Build history of the part. All positions in model axes, mm. Face numbers are marked on the shaded views. A direction names the side the tool comes from. Give positions to 0.01 mm unless a question says otherwise; leave off trailing zeros. Order: outer loops, then holes, each group sorted by start corner. A loop starts at its lowest first (then second) coordinate and runs counter-clockwise, first axis right, second up. Notation, with made-up numbers: (-14, 61.25) -> (24, 61.25) arc R18 cw to (24, 93.25) -> close; hole circle Ø2 at (13.25, 27.5). An arc over 180 degrees is marked (long way). Use a Markdown table: item, result. Add a question column.
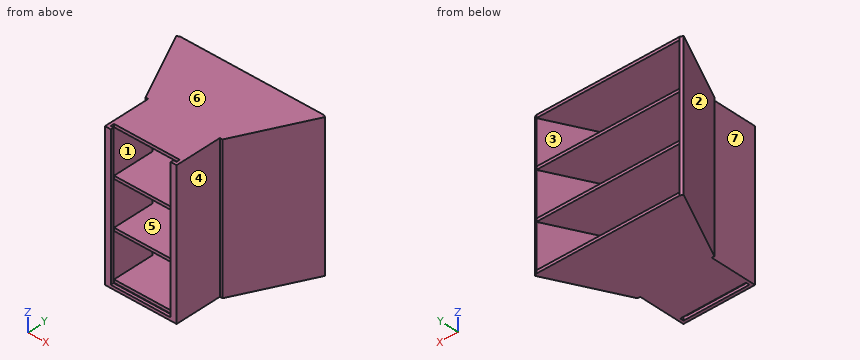
Autodesk Inventor part; units mm, degrees
ref_plane "YZ Plane" through (0, 0, 0) normal (1, 0, 0) x (0, 1, 0)
ref_plane "XZ Plane" through (0, 0, 0) normal (0, 1, 0) x (-1, 0, 0)
ref_plane "XY Plane" through (0, 0, 0) normal (0, 0, 1) x (1, 0, 0)
sketch "Sketch1" plane through (0, 0, 0) normal (0, 1, 0) x (-1, 0, 0)
  line L0 (0, 0) -> (-76.2, 0)
  line L1 (-76.2, 0) -> (-76.2, 152.4)
  line L2 (-76.2, 152.4) -> (0, 152.4)
  line L3 (0, 152.4) -> (0, 0)
  line L4 (-3.175, 149.225) -> (-73.025, 149.225)
  line L5 (-73.025, 149.225) -> (-73.025, 3.175)
  line L6 (-73.025, 3.175) -> (-3.175, 3.175)
  line L7 (-3.175, 3.175) -> (-3.175, 149.225)
  dimension "d0" = 76.2
  dimension "d1" = 152.4
  dimension "d2" = 3.175
extrude "Extrusion1" add sketch "Sketch1" along normal blind 43.815
sketch "Sketch2" plane through (0, 0, 0) normal (0, -1, 0) x (1, 0, 0)
  line L0 (0, 152.4) -> (76.2, 152.4)
  line L1 (76.2, 0) -> (0, 0)
  line L2 (76.2, 152.4) -> (73.025, 152.4)
  line L3 (73.025, 152.4) -> (73.025, 0)
  line L4 (73.025, 0) -> (76.2, 0)
  line L5 (76.2, 0) -> (76.2, 152.4)
  line L6 (0, 0) -> (3.175, 0)
  line L7 (3.175, 0) -> (3.175, 152.4)
  line L8 (3.175, 152.4) -> (0, 152.4)
  line L9 (0, 152.4) -> (0, 0)
  dimension "d5" = 3.175
  dimension "d6" = 3.175
extrude "Extrusion2" add sketch "Sketch2" along normal blind 3.81 contours L0 L7 L1 L9 | L0 L5 L1 L3
sketch "Sketch3" plane through (0, -3.81, 0) normal (0, -1, 0) x (1, 0, 0)
  line L0 (0, 152.4) -> (76.2, 152.4)
  line L1 (76.2, 0) -> (0, 0)
  line L2 (76.2, 152.4) -> (69.85, 152.4)
  line L3 (69.85, 152.4) -> (69.85, 0)
  line L4 (69.85, 0) -> (76.2, 0)
  line L5 (76.2, 0) -> (76.2, 152.4)
  line L6 (0, 152.4) -> (6.35, 152.4)
  line L7 (6.35, 152.4) -> (6.35, 0)
  line L8 (6.35, 0) -> (0, 0)
  line L9 (0, 0) -> (0, 152.4)
  dimension "d9" = 6.35
  dimension "d10" = 6.35
extrude "Extrusion3" add sketch "Sketch3" along normal blind 3.175 contours L0 L7 L1 L9 | L0 L5 L1 L3
sketch "Sketch4" plane through (73.025, 0, 0) normal (0, 0, -1) x (-1, 0, 0)
  line L0 (0, -3.81) -> (3.175, -3.81)
  line L1 (73.025, -6.985) -> (66.675, -6.985)
  line L2 (3.175, -3.81) -> (66.675, -3.81)
  line L3 (66.675, -3.81) -> (66.675, -6.985)
  line L4 (66.675, -6.985) -> (3.175, -6.985)
  line L5 (3.175, -6.985) -> (3.175, -3.81)
  point P0 (73.025, 0)
extrude "Extrusion4" add sketch "Sketch4" against normal blind 3.175
sketch "Sketch5" plane through (3.175, 0, 3.175) normal (1, 0, 0) x (0, 0, -1)
  line L0 (-146.05, 0) -> (-146.05, 43.815) construction
  line L1 (-146.05, 43.815) -> (-99.568, 43.815) construction
  line L2 (-146.05, 43.815) -> (0, 43.815) construction
  line L3 (-99.568, 43.815) -> (-96.393, 43.815) construction
  line L4 (-96.393, 43.815) -> (-49.657, 43.815) construction
  line L5 (-49.657, 43.815) -> (-46.482, 43.815) construction
  line L6 (0, 0) -> (0, 43.815) construction
  line L7 (-46.482, 43.815) -> (0, 43.815) construction
  line L8 (-46.482, 43.815) -> (0, 43.815) construction
  line L9 (-46.482, 43.815) -> (0, 43.815) construction
  line L10 (-99.568, 43.815) -> (-96.393, 43.815)
  line L11 (-96.393, 43.815) -> (-96.393, 0)
  line L12 (-96.393, 0) -> (-99.568, 0)
  line L13 (-99.568, 0) -> (-99.568, 43.815)
  line L14 (-49.657, 43.815) -> (-46.482, 43.815)
  line L15 (-46.482, 43.815) -> (-46.482, 0)
  line L16 (-46.482, 0) -> (-49.657, 0)
  line L17 (-49.657, 0) -> (-49.657, 43.815)
  point P0 (3.175, 0)
  dimension "d15" = 46.482
  dimension "d16" = 3.175
  dimension "d17" = 46.736
  dimension "d18" = 3.175
  dimension "d19" = 43.815
  dimension "d20" = 43.815
extrude "Extrusion5" add sketch "Sketch5" along normal up to next
sketch "Sketch6" plane through (3.175, 0, 152.4) normal (0, 0, 1) x (1, 0, 0)
  line L0 (73.025, 43.815) -> (-3.175, 43.815)
  line L1 (-3.175, 43.815) -> (73.025, 43.815)
  line L2 (73.025, 43.815) -> (73.025, 120.015)
  line L3 (73.025, 120.015) -> (-3.175, 120.015)
  line L4 (-3.175, 120.015) -> (-3.175, 43.815)
  point P0 (-3.175, 0)
  dimension "d23" = 76.2
extrude "Extrusion6" add sketch "Sketch6" against normal blind 3.175
sketch "Sketch7" plane through (3.175, 0, 152.4) normal (0, 0, 1) x (1, 0, 0)
  line L0 (73.025, 120.015) -> (73.025, 43.815)
  line L1 (73.025, 120.015) -> (111.125, 120.015)
  line L2 (73.025, 43.815) -> (111.125, 120.015)
  line L3 (73.025, 120.015) -> (-3.175, 120.015)
  line L4 (-3.175, 120.015) -> (-41.275, 120.015)
  line L5 (-3.175, 120.015) -> (34.925, 120.015) construction
  line L6 (-3.175, 43.815) -> (-3.175, 120.015)
  line L7 (-41.275, 120.015) -> (-3.175, 43.815)
  point P0 (-3.175, 0)
  dimension "d26" = 38.1
  dimension "d27" = 38.1
  dimension "d28" = 180
extrude "Extrusion7" add sketch "Sketch7" against normal blind 3.175
sketch "Sketch8" plane through (76.2, 43.815, 0) normal (0, 0, -1) x (-1, 0, 0)
  line L0 (3.175, 0) -> (0, 0)
  line L1 (0, 0) -> (-38.1, 76.2)
  line L2 (114.3, 76.2) -> (-38.1, 76.2)
  line L3 (-38.1, 76.2) -> (114.3, 76.2)
  line L4 (76.2, 0) -> (73.025, 0)
  line L5 (114.3, 76.2) -> (76.2, 0)
  line L6 (0, 0) -> (76.2, 0)
  line L7 (73.025, 0) -> (3.175, 0)
  point P0 (76.2, -43.815)
extrude "Extrusion8" add sketch "Sketch8" against normal blind 3.175
sketch "Sketch9" plane through (76.2, 43.815, 152.4) normal (0.8944, -0.4472, 0) x (0, 0, -1)
  line L0 (0, 85.1942) -> (3.175, 85.1942)
  line L1 (152.4, 85.1942) -> (152.4, 0)
  line L2 (0, 85.1942) -> (152.4, 85.1942)
  line L3 (152.4, 85.1942) -> (152.4, 0)
  line L4 (152.4, 0) -> (0, 0)
  line L5 (0, 0) -> (0, 85.1942)
  point P0 (152.4, -73.267)
extrude "Extrusion9" add sketch "Sketch9" along normal blind 3.175
sketch "Sketch10" plane through (0, 43.815, 0) normal (-0.8944, -0.4472, 0) x (0, 0, 1)
  line L0 (0, 85.1942) -> (3.175, 85.1942)
  line L1 (152.4, -45.4369) -> (152.4, 0)
  line L2 (0, 85.1942) -> (152.4, 85.1942)
  line L3 (152.4, 85.1942) -> (152.4, 0)
  line L4 (152.4, 0) -> (0, 0)
  line L5 (0, 0) -> (0, 85.1942)
  point P0 (0, -39.1893)
extrude "Extrusion10" add sketch "Sketch10" along normal blind 3.175
sketch "Sketch11" plane through (114.3, 120.015, 152.4) normal (0, 1, 0) x (1, 0, 0)
  line L0 (-111.125, 49.657) -> (-41.275, 49.657) construction
  line L1 (-111.125, 49.657) -> (-152.4, 49.657) construction
  line L2 (-152.4, 3.175) -> (-152.4, 149.225) construction
  line L3 (-111.125, 52.832) -> (-41.275, 52.832) construction
  line L4 (-41.275, 52.832) -> (0, 52.832) construction
  line L5 (0, 149.225) -> (0, 3.175) construction
  line L6 (-111.125, 99.568) -> (-41.275, 99.568) construction
  line L7 (-111.125, 99.568) -> (-152.4, 99.568) construction
  line L8 (-111.125, 102.743) -> (-41.275, 102.743) construction
  line L9 (-41.275, 102.743) -> (0, 102.743) construction
  line L10 (-152.4, 49.657) -> (0, 49.657)
  line L11 (0, 49.657) -> (0, 52.832)
  line L12 (0, 52.832) -> (-152.4, 52.832)
  line L13 (-152.4, 52.832) -> (-152.4, 49.657)
  line L14 (-152.4, 99.568) -> (0, 99.568)
  line L15 (0, 99.568) -> (0, 102.743)
  line L16 (0, 102.743) -> (-152.4, 102.743)
  line L17 (-152.4, 102.743) -> (-152.4, 99.568)
  point P0 (-114.3, 152.4)
extrude "Extrusion11" add sketch "Sketch11" against normal blind 3.175
sketch "Sketch12" plane through (-38.1, 120.015, 102.743) normal (0, 0, 1) x (1, 0, 0)
  line L0 (150.8125, -3.175) -> (1.5875, -3.175)
  line L1 (1.5875, -3.175) -> (38.1, -76.2)
  line L2 (38.1, -76.2) -> (114.3, -76.2)
  line L3 (152.4, 0) -> (150.8125, -3.175)
  line L4 (114.3, -76.2) -> (150.8125, -3.175)
  line L5 (150.8125, -3.175) -> (1.5875, -3.175)
  point P0 (38.1, -120.015)
extrude "Extrusion12" add sketch "Sketch12" against normal blind 3.175
sketch "Sketch13" plane through (-38.1, 120.015, 52.832) normal (0, 0, 1) x (1, 0, 0)
  line L0 (150.8125, -3.175) -> (1.5875, -3.175)
  line L1 (1.5875, -3.175) -> (38.1, -76.2)
  line L2 (38.1, -76.2) -> (114.3, -76.2)
  line L3 (152.4, 0) -> (150.8125, -3.175)
  line L4 (114.3, -76.2) -> (150.8125, -3.175)
  line L5 (150.8125, -3.175) -> (1.5875, -3.175)
  point P0 (38.1, -120.015)
extrude "Extrusion13" add sketch "Sketch13" against normal blind 3.175
sketch "Sketch14" plane through (3.175, 0, 152.4) normal (0, 0, 1) x (1, 0, 0)
  line L0 (-3.175, 43.815) -> (-6.0148, 42.3951)
  line L1 (-6.0148, 42.3951) -> (-3.175, 42.3951)
  line L2 (-3.175, 43.815) -> (-3.175, -6.985)
  line L3 (-3.175, 42.3951) -> (-3.175, 43.815)
  line L4 (-3.175, 43.815) -> (-6.0148, 42.3951)
  line L5 (75.8648, 42.3951) -> (73.025, 42.3951)
  line L6 (73.025, -6.985) -> (73.025, 43.815)
  line L7 (73.025, 42.3951) -> (73.025, 43.815)
  line L8 (73.025, 43.815) -> (75.8648, 42.3951)
  line L9 (73.025, 43.815) -> (75.8648, 42.3951)
  point P0 (-3.175, 0)
extrude "Extrusion14" add sketch "Sketch14" against normal blind 152.4
properties part number "BeadCompartments_3"
(1) Pin check, flat tips, straight feed: pin 1 Ø1 at (y, z) = (106.5, 82.5) entering from +X; pin 2 Ø5 at (x, y) = (80, 27.5) entering from -Z; pin 3 Ø8 at (x, z) = (76.5, 62) entering from -Y (3 decimals); pin 4 Ø10 at (y, z) = (18, 105) entering from -X. Stop position of each tip, or through.
(2) Band-saw the part on B-B on y = 15.5. Give the cut face in (x, z) (3 decimals).
(3) Band-saw the part on A-A on x = 27.5. Give the cut face in (y, z) (3 decimals), plus the area to 3 significant figures.
(4) Mould opens along X. For the marked faces 1, 2, 3 and 4 say: released by +X, released by -X, zero draft, split by the parting line, or undercut.
(5) Band-saw the part on D-D on y = 50. Give the cut face in (x, z) (1 decimal).
(6) Wall check: probe 1 along Z at (x, y) = (98.5, 94.5) (3 decimals); probe 2 along X at (y, z) = (4, 84.5) (3 decimals); probe 3 along X at (y, z) = (95, 104). Give the ranges that are in metal, low to high.
(7) Band-saw the part on C-C on z = 15.5. Give the cut face in (x, y) (3 decimals).
(8) Tool access for the marked faces 5, 6 and 7: list every direction of +Z, -Z, +X, -X, +Y, -Y with a clear straight run to the whole face (end or side of a thin tool).
Response:
| question | item | result |
|---|---|---|
| 1 | pin 1 | stops at x = 111.34 |
| 1 | pin 2 | passes through |
| 1 | pin 3 | stops at y = -6.985 |
| 1 | pin 4 | stops at x = 0 |
| 2 | outline | (0, 0) -> (76.2, 0) -> (76.2, 152.4) -> (0, 152.4) -> close; hole (3.175, 3.175) -> (73.025, 3.175) -> (73.025, 49.657) -> (3.175, 49.657) -> close; hole (3.175, 52.832) -> (73.025, 52.832) -> (73.025, 99.568) -> (3.175, 99.568) -> close; hole (3.175, 102.743) -> (73.025, 102.743) -> (73.025, 149.225) -> (3.175, 149.225) -> close |
| 3 | outline | (-6.985, 0) -> (-3.81, 0) -> (-3.81, 3.175) -> (-6.985, 3.175) -> close; (0, 0) -> (120.015, 0) -> (120.015, 3.175) -> (0, 3.175) -> close; (0, 49.657) -> (120.015, 49.657) -> (120.015, 52.832) -> (0, 52.832) -> close; (0, 99.568) -> (120.015, 99.568) -> (120.015, 102.743) -> (0, 102.743) -> close; (0, 149.225) -> (120.015, 149.225) -> (120.015, 152.4) -> (0, 152.4) -> close |
| 3 | area | 1,530 mm² |
| 4 | face 1 | undercut |
| 4 | face 2 | released by -X |
| 4 | face 3 | undercut |
| 4 | face 4 | released by +X |
| 5 | outline | (-6.6, 0) -> (82.8, 0) -> (82.8, 152.4) -> (-6.6, 152.4) -> close; hole (-3.1, 3.2) -> (79.3, 3.2) -> (79.3, 49.7) -> (-3.1, 49.7) -> close; hole (-3.1, 52.8) -> (79.3, 52.8) -> (79.3, 99.6) -> (-3.1, 99.6) -> close; hole (-3.1, 102.7) -> (79.3, 102.7) -> (79.3, 149.2) -> (-3.1, 149.2) -> close |
| 6 | probe 1 | z = 0 to 3.175, 49.657 to 52.832, 99.568 to 102.743, 149.225 to 152.4 |
| 6 | probe 2 | x = 0 to 3.175, 73.025 to 76.2 |
| 6 | probe 3 | x = -29.14 to -25.59, 101.79 to 105.34 |
| 7 | outline | (-40.94, 118.595) -> (-2.84, 42.395) -> (0, 42.395) -> (0, -6.985) -> (6.35, -6.985) -> (6.35, -3.81) -> (3.175, -3.81) -> (3.175, 43.815) -> (0, 43.815) -> (-38.1, 120.015) -> close; (69.85, -6.985) -> (76.2, -6.985) -> (76.2, 42.395) -> (79.04, 42.395) -> (117.14, 118.595) -> (114.3, 120.015) -> (76.2, 43.815) -> (73.025, 43.815) -> (73.025, -3.81) -> (69.85, -3.81) -> close |
| 8 | face 5 | +Y |
| 8 | face 6 | +Z, +X, -X, +Y, -Y |
| 8 | face 7 | +Z, -Z, -X, -Y |
